from build123d import *

# Parameters (mm, degrees)
BOSS_EXTRUDE1_DEPTH              = 5
SKETCH3_W                        = 11
SKETCH3_H                        = 5
BOSS_EXTRUDE2_DEPTH              = 5
SKETCH4_W                        = 5
SKETCH4_H                        = 5
BOSS_EXTRUDE3_DEPTH              = 21
SKETCH5_W                        = 10
SKETCH5_H                        = 5
BOSS_EXTRUDE4_DEPTH              = 20
SKETCH6_W                        = 11
SKETCH6_H                        = 5
BOSS_EXTRUDE5_DEPTH              = 5
SKETCH7_W                        = 5
SKETCH7_H                        = 5
BOSS_EXTRUDE6_DEPTH              = 21
SKETCH8_W                        = 10
SKETCH8_H                        = 5
BOSS_EXTRUDE7_DEPTH              = 20
SKETCH11_W                       = 10
SKETCH11_H                       = 5
BOSS_EXTRUDE8_DEPTH              = 3.5
SKETCH12_W                       = 10
SKETCH12_H                       = 5
BOSS_EXTRUDE9_DEPTH              = 3.5
CUT_EXTRUDE6_DEPTH               = 14.5
CUT_EXTRUDE8_DEPTH               = 41.078048855
CUT_EXTRUDE8_DEPTH_BACK          = 14.5
SKETCH17_W                       = 1.38
SKETCH17_H                       = 3.56
CUT_EXTRUDE9_DEPTH               = 14.5
CUT_EXTRUDE10_DEPTH              = 14.5
SKETCH_1_W                       = 8
SKETCH_1_H                       = 25
EXTRUDE_1_DEPTH                  = 5
SKETCH_2_W                       = 8
SKETCH_2_H                       = 25
EXTRUDE_2_DEPTH                  = 5
AUFSATZ_LINEAR_AUSTRAGEN1_DEPTH  = 4
SKIZZE3_W                        = 10
SKIZZE3_H                        = 5
SCHNITT_LINEAR_AUSTRAGEN2_DEPTH  = 3.5
SCHNITT_LINEAR_AUSTRAGEN3_DEPTH  = 4
AUFSATZ_LINEAR_AUSTRAGEN3_DEPTH  = 11
SKIZZE7_R                        = 1.5
SCHNITT_LINEAR_AUSTRAGEN6_DEPTH  = 10
SKIZZE8_W                        = 10
SKIZZE8_H                        = 5
SCHNITT_LINEAR_AUSTRAGEN8_DEPTH  = 4
AUFSATZ_LINEAR_AUSTRAGEN4_DEPTH  = 4
SCHNITT_LINEAR_AUSTRAGEN9_DEPTH  = 4
AUFSATZ_LINEAR_AUSTRAGEN6_DEPTH  = 11
SKIZZE12_R                       = 1.5
SCHNITT_LINEAR_AUSTRAGEN10_DEPTH = 11
SKIZZE15_W                       = 8
SKIZZE15_H                       = 20
SCHNITT_LINEAR_AUSTRAGEN11_DEPTH = 37
AUFSATZ_LINEAR_AUSTRAGEN7_DEPTH  = 20
AUFSATZ_LINEAR_AUSTRAGEN8_DEPTH  = 20
SKIZZE18_W                       = 2.855193512
SKIZZE18_H                       = 5
SCHNITT_LINEAR_AUSTRAGEN12_DEPTH = 35


with BuildPart() as part:
    # Sketch1 → Boss-Extrude1 (new body)
    with BuildSketch(Plane(origin=(0, 0, 0), x_dir=(1, 0, 0), z_dir=(0, 1, 0))):
        Polygon((5.5, 3), (5.5, 0), (5.5, -3), (5.5, -8.5), (0, -8.5), (-5.5, -8.5), (-5.5, -3), (-5.5, 8.5), (0, 8.5), (5.5, 8.5), align=None)
    extrude(amount=BOSS_EXTRUDE1_DEPTH)

    # Sketch3 → Boss-Extrude2 (add)
    with BuildSketch(Plane.XY.offset(8.5)):
        with Locations((0, 2.5)):
            Rectangle(SKETCH3_W, SKETCH3_H)
    extrude(amount=BOSS_EXTRUDE2_DEPTH)

    # Sketch4 → Boss-Extrude3 (add)
    with BuildSketch(Plane(origin=(5.5, 0, 0), x_dir=(0, 0, -1), z_dir=(1, 0, 0))):
        with Locations((-11, 2.5)):
            Rectangle(SKETCH4_W, SKETCH4_H)
    extrude(amount=BOSS_EXTRUDE3_DEPTH)

    # Sketch5 → Boss-Extrude4 (add)
    with BuildSketch(Plane.XZ):
        with Locations((21.5, 11)):
            Rectangle(SKETCH5_W, SKETCH5_H)
    extrude(amount=BOSS_EXTRUDE4_DEPTH)

    # Sketch6 → Boss-Extrude5 (add)
    with BuildSketch(Plane(origin=(0, 0, -8.5), x_dir=(-1, 0, 0), z_dir=(0, 0, -1))):
        with Locations((0, 2.5)):
            Rectangle(SKETCH6_W, SKETCH6_H)
    extrude(amount=BOSS_EXTRUDE5_DEPTH)

    # Sketch7 → Boss-Extrude6 (add)
    with BuildSketch(Plane(origin=(5.5, 0, 0), x_dir=(0, 0, -1), z_dir=(1, 0, 0))):
        with Locations((11, 2.5)):
            Rectangle(SKETCH7_W, SKETCH7_H)
    extrude(amount=BOSS_EXTRUDE6_DEPTH)

    # Sketch8 → Boss-Extrude7 (add)
    with BuildSketch(Plane(origin=(0, 0, 0), x_dir=(-1, 0, 0), z_dir=(0, -1, 0))):
        with Locations((-21.5, 11)):
            Rectangle(SKETCH8_W, SKETCH8_H)
    extrude(amount=BOSS_EXTRUDE7_DEPTH)

    # Sketch11 → Boss-Extrude8 (add)
    with BuildSketch(Plane(origin=(0, 0, 8.5), x_dir=(-1, 0, 0), z_dir=(0, 0, -1))):
        with Locations((-21.5, -12.5)):
            Rectangle(SKETCH11_W, SKETCH11_H)
    extrude(amount=BOSS_EXTRUDE8_DEPTH)

    # Sketch12 → Boss-Extrude9 (add)
    with BuildSketch(Plane.XY.offset(-8.5)):
        with Locations((21.5, -12.5)):
            Rectangle(SKETCH12_W, SKETCH12_H)
    extrude(amount=BOSS_EXTRUDE9_DEPTH)

    # Sketch14 → Cut-Extrude6 (cut)
    with BuildSketch(Plane(origin=(26.5, 0, 0), x_dir=(0, 0, -1), z_dir=(1, 0, 0))):
        Polygon((-6.379568334, -12.879568334), (-6.379568334, -15), (-5, -15), (-5, -11.439784167), (-6.379568334, -11.439784167), align=None)
    extrude(amount=-CUT_EXTRUDE6_DEPTH, mode=Mode.SUBTRACT)

    # Sketch16 → Cut-Extrude8 (cut, two sides: drawn at the far end of the back side and taken through both)
    with BuildSketch(Plane(origin=(26.5, 0, 0), x_dir=(0, 0, -1), z_dir=(1, 0, 0)).offset(-CUT_EXTRUDE8_DEPTH_BACK)):
        Polygon((-6.379568334, -13), (-8.5, -15), (-7.439784167, -15), (-6.379568334, -15), align=None)
    extrude(amount=CUT_EXTRUDE8_DEPTH + CUT_EXTRUDE8_DEPTH_BACK, mode=Mode.SUBTRACT)

    # Sketch17 → Cut-Extrude9 (cut)
    with BuildSketch(Plane(origin=(26.5, 0, 0), x_dir=(0, 0, -1), z_dir=(1, 0, 0))):
        with Locations((5.69, -13.22)):
            Rectangle(SKETCH17_W, SKETCH17_H)
    extrude(amount=-CUT_EXTRUDE9_DEPTH, mode=Mode.SUBTRACT)

    # Sketch18 → Cut-Extrude10 (cut)
    with BuildSketch(Plane(origin=(26.5, 0, 0), x_dir=(0, 0, -1), z_dir=(1, 0, 0))):
        Polygon((6.38, -13), (6.38, -15), (8.5, -15), align=None)
    extrude(amount=-CUT_EXTRUDE10_DEPTH, mode=Mode.SUBTRACT)

    # 草图1 → 凸台-拉伸1 (add)
    with BuildSketch(Plane.XY.offset(13.5)):
        with Locations((30.5, -7.5)):
            Rectangle(SKETCH_1_W, SKETCH_1_H)
    extrude(amount=-EXTRUDE_1_DEPTH)

    # 草图2 → 凸台-拉伸2 (add)
    with BuildSketch(Plane(origin=(0, 0, -13.5), x_dir=(-1, 0, 0), z_dir=(0, 0, -1))):
        with Locations((-30.5, -7.5)):
            Rectangle(SKETCH_2_W, SKETCH_2_H)
    extrude(amount=-EXTRUDE_2_DEPTH)

    # Skizze2 → Aufsatz-Linear austragen1 (add)
    with BuildSketch(Plane.XY.offset(13.5)):
        Polygon((-5.5, 5), (-5.5, 0), (16.5, 0), (16.5, -20), (34.5, -20), (34.5, 5), align=None)
    extrude(amount=AUFSATZ_LINEAR_AUSTRAGEN1_DEPTH)

    # Skizze3 → Schnitt-Linear austragen2 (cut)
    with BuildSketch(Plane(origin=(0, 0, 5), x_dir=(-1, 0, 0), z_dir=(0, 0, -1))):
        with Locations((-21.5, -12.5)):
            Rectangle(SKIZZE3_W, SKIZZE3_H)
    extrude(amount=-SCHNITT_LINEAR_AUSTRAGEN2_DEPTH, mode=Mode.SUBTRACT)

    # Skizze4 → Schnitt-Linear austragen3 (cut)
    with BuildSketch(Plane(origin=(0, 0, 8.5), x_dir=(-1, 0, 0), z_dir=(0, 0, -1))):
        Polygon((-34.5, 5), (-34.5, -20), (-16.5, -20), (-16.5, 0), (-5.5, 0), (-5.5, 5), align=None)
    extrude(amount=-SCHNITT_LINEAR_AUSTRAGEN3_DEPTH, mode=Mode.SUBTRACT)

    # Skizze6 → Aufsatz-Linear austragen3 (add)
    with BuildSketch(Plane.XY.offset(17.5)):
        Polygon((16, 5), (11, 5), (11, 0), (16.5, 0), (21, 0), (21, 5), align=None)
    extrude(amount=AUFSATZ_LINEAR_AUSTRAGEN3_DEPTH)

    # Skizze7 → Schnitt-Linear austragen6 (cut)
    with BuildSketch(Plane(origin=(0, 5, 0), x_dir=(1, 0, 0), z_dir=(0, 1, 0))):
        with Locations(Location((16, -23, 0), (0, 0, 270))):
            Circle(SKIZZE7_R)
    extrude(amount=-SCHNITT_LINEAR_AUSTRAGEN6_DEPTH, mode=Mode.SUBTRACT)

    # Skizze8 → Schnitt-Linear austragen8 (cut)
    with BuildSketch(Plane.XY.offset(-8.5)):
        with Locations((21.5, -12.5)):
            Rectangle(SKIZZE8_W, SKIZZE8_H)
    extrude(amount=SCHNITT_LINEAR_AUSTRAGEN8_DEPTH, mode=Mode.SUBTRACT)

    # Skizze9 → Aufsatz-Linear austragen4 (add)
    with BuildSketch(Plane(origin=(0, 0, -13.5), x_dir=(-1, 0, 0), z_dir=(0, 0, -1))):
        Polygon((-34.5, 5), (-34.5, -20), (-16.5, -20), (-16.5, 0), (5.5, 0), (5.5, 5), align=None)
    extrude(amount=AUFSATZ_LINEAR_AUSTRAGEN4_DEPTH)

    # Skizze10 → Schnitt-Linear austragen9 (cut)
    with BuildSketch(Plane.XY.offset(-8.5)):
        Polygon((5.5, 5), (5.5, 0), (16.5, 0), (16.5, -20), (34.5, -20), (34.5, 5), align=None)
    extrude(amount=-SCHNITT_LINEAR_AUSTRAGEN9_DEPTH, mode=Mode.SUBTRACT)

    # Skizze11 → Aufsatz-Linear austragen6 (add)
    with BuildSketch(Plane(origin=(0, 0, -17.5), x_dir=(-1, 0, 0), z_dir=(0, 0, -1))):
        Polygon((-11, 0), (-11, 5), (-21, 5), (-21, 0), (-16.5, 0), align=None)
    extrude(amount=AUFSATZ_LINEAR_AUSTRAGEN6_DEPTH)

    # Skizze12 → Schnitt-Linear austragen10 (cut)
    with BuildSketch(Plane(origin=(0, 5, 0), x_dir=(1, 0, 0), z_dir=(0, 1, 0))):
        with Locations(Location((16, 23, 0), (0, 0, 270))):
            Circle(SKIZZE12_R)
    extrude(amount=-SCHNITT_LINEAR_AUSTRAGEN10_DEPTH, mode=Mode.SUBTRACT)

    # Skizze15 → Schnitt-Linear austragen11 (cut)
    with BuildSketch(Plane.XY.offset(17.5)):
        with Locations((20.5, -10)):
            Rectangle(SKIZZE15_W, SKIZZE15_H)
    extrude(amount=-SCHNITT_LINEAR_AUSTRAGEN11_DEPTH, mode=Mode.SUBTRACT)

    # Skizze16 → Aufsatz-Linear austragen7 (add)
    with BuildSketch(Plane.XZ):
        Polygon((7.355193512, 12.5), (7.355193512, 17.5), (-2.644806488, 17.5), (-2.644806488, 12.5), (5.5, 12.5), align=None)
    extrude(amount=AUFSATZ_LINEAR_AUSTRAGEN7_DEPTH)

    # Skizze17 → Aufsatz-Linear austragen8 (add)
    with BuildSketch(Plane.XZ):
        Polygon((5.5, -12.5), (-2.644806488, -12.5), (-2.644806488, -17.5), (7.355193512, -17.5), (7.355193512, -12.5), align=None)
    extrude(amount=AUFSATZ_LINEAR_AUSTRAGEN8_DEPTH)

    # Skizze18 → Schnitt-Linear austragen12 (cut)
    with BuildSketch(Plane(origin=(0, 0, -17.5), x_dir=(-1, 0, 0), z_dir=(0, 0, -1))):
        with Locations((4.072403244, 2.5)):
            Rectangle(SKIZZE18_W, SKIZZE18_H)
    extrude(amount=-SCHNITT_LINEAR_AUSTRAGEN12_DEPTH, mode=Mode.SUBTRACT)


solid = part.part
CAD build for the part. Positions are in the model's coordinates, mm. A direction names the side the tool comes from. Coordinates: 2 decimals unless noted, no trailing zeros. Loops run counter-clockwise (first coordinate to the right, second up) from the corner with the lowest first, then second, coordinate; pieces in that order, holes last. Notation, with made-up numbers: (-38, 61.25) - (15, 61.25) arc R27 cw to (15, 90.25) - close; hole circle Ø2 at (26, -33). An arc over 180 degrees is marked (long way). Use one line per item in the form item = value. Start each with the question number.
1) Tool access for faces 1 (the face through (21, 2, 23)), 2 (the face through (3, -7, 17.5)), 3 (the face through (5.5, 2, 0)): list every direction of +Z, -Z, +X, -X, +Y, -Y with a clear straight run to the whole face (end or side of a thin tool).
2) Band-saw the part on D-D (y = -17.25). Give the cut face in (x, z).
3) Two-plate mould, pull along X, no slides. Class faces 4 (the face through (3, -7, -17.5)), 5 (the face through (24.5, -10, -15)), 6 (the face through (-2.645, 1, 0)): +X half, -X half, draft (parallel to the pull), parting line (faces both ways), or undercut.
4) Flat gauge pins, fed straight in: pin 1 (11 mm diameter, centred on x = 30, y = -11.5, fed in from +Z); pin 2 (1 mm diameter, centred on x = 22, y = -2, fed in from -Z); pin 3 (1.5 mm diameter, centred on y = 3, z = 25.5, fed in from +X); pin 4 (9 mm diameter, centred on x = -0.5, z = -1, fed in from -Y). Where does each tip first touch, or does it go through?
5) Drill centre lines: L1, parallel to Z at x = 28, y = 3; L2, parallel to X at y = 2.2, z = 23; L3, parallel to X at y = 0.25, z = 1.5. Where is each one in solid material? Low to high. Write a range as from..to.
6) Band-saw the part on B-B (x = 19). Give the cut face in (y, z).
7) Band-saw the part on C-C (z = 23). Give the cut face in (x, y).
8) Band-saw the part on A-A (y = 1.25). Give the cut face in (x, z), and give its area (3 significant figures).
Check values:
q1.face_1 = +Z, +X, +Y, -Y
q1.face_2 = +Z, -X, +Y, -Y
q1.face_3 = +X, +Y, -Y
q2.outline = (-2.64, -17.5) - (7.36, -17.5) - (7.36, -12.5) - (-2.64, -12.5) - close; (-2.64, 12.5) - (7.36, 12.5) - (7.36, 17.5) - (-2.64, 17.5) - close; (24.5, -17.5) - (34.5, -17.5) - (34.5, -12.5) - (24.5, -12.5) - close; (24.5, 12.5) - (34.5, 12.5) - (34.5, 17.5) - (24.5, 17.5) - close
q3.face_4 = draft
q3.face_5 = undercut
q3.face_6 = -X half
q4.pin_1 = 17.5
q4.pin_2 = through
q4.pin_3 = 21
q4.pin_4 = 0
q5.L1 = -17.5..-12.5, 12.5..17.5
q5.L2 = 11..14.5, 17.5..21
q5.L3 = -2.64..5.5
q6.outline = (0, -28.5) - (5, -28.5) - (5, -12.5) - (0, -12.5) - close; (0, 12.5) - (5, 12.5) - (5, 28.5) - (0, 28.5) - close
q7.outline = (11, 0) - (14.5, 0) - (14.5, 5) - (11, 5) - close; (17.5, 0) - (21, 0) - (21, 5) - (17.5, 5) - close
q8.outline = (-2.64, -17.5) - (11, -17.5) - (11, -28.5) - (21, -28.5) - (21, -17.5) - (34.5, -17.5) - (34.5, -12.5) - (5.5, -12.5) - (5.5, 12.5) - (34.5, 12.5) - (34.5, 17.5) - (21, 17.5) - (21, 28.5) - (11, 28.5) - (11, 17.5) - (-2.64, 17.5) - close; hole circle Ø3 at (16, -23); hole circle Ø3 at (16, 23)
q8.area = 781 mm2
